Job drawing, mm, ordinate dimensions from the low corner. One solid piece. A direction names the side the tool comes from. Round coordinates to 2 decimals unless told otherwise and drop trailing zeros. Loops run counter-clockwise (first coordinate to the right, second up) from the corner with the lowest first, then second, coordinate; pieces in that order, holes last. Notation, with made-up numbers: M -37.75,-26 L -23.75,-26 A26 cw -23.75,13 Z; hole C 39,-40 d1. An arc over 180 degrees is marked long. One line per item, written item: value.
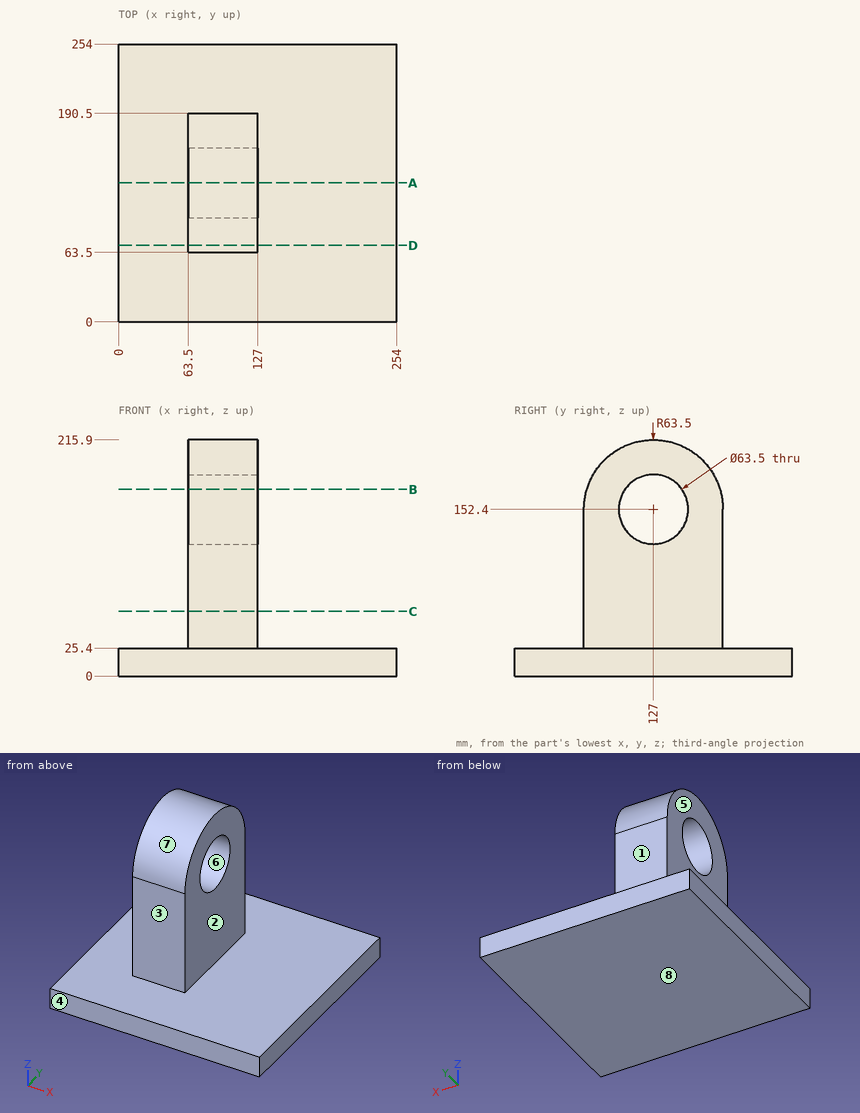
Item 1: Wall check: line 1 along Z through (x, y) = (89, 127); line 2 along Y through (x, z) = (83, 152); line 3 along X through (y, z) = (100.5, 58.5). Give the ranges that are in metal, low to high.
Check values:
line 1: z = 0 to 120.65, 184.15 to 215.9
line 2: y = 63.5 to 95.25, 158.75 to 190.5
line 3: x = 63.5 to 127
Item 2: Which spindle directions (+Z, -Z, +X, -X, +Y, -Y) get a long thin tool onto all of the face, cutting with end or side? Do the marked faces 1, 2, 3 and 4. Say none if no direction does.
Check values:
face 1: +Z, +X, -X, +Y
face 2: +Z, +X, +Y, -Y
face 3: +Z, +X, -X, -Y
face 4: +Z, -Z, +X, -X, -Y
Item 3: Slice it at A-A, the plane y = 127. Give the cut face in (x, z).
Check values:
outline: M 0,0 L 254,0 L 254,25.4 L 127,25.4 L 127,120.65 L 63.5,120.65 L 63.5,25.4 L 0,25.4 Z; M 63.5,184.15 L 127,184.15 L 127,215.9 L 63.5,215.9 Z
Item 4: Slice it at C-C, the plane z = 59. Give the cut face in (x, y), and give its area (3 significant figures).
Check values:
outline: M 63.5,63.5 L 127,63.5 L 127,190.5 L 63.5,190.5 Z
area: 8,060 mm2
Item 5: Drop flat-ended pins along their axis: P1, Ø2, axis at y = 171.5, z = 77.5, coming from the -X side; P2, Ø4, axis at y = 164.5, z = 161.5, coming from the +X side; P3, Ø6, axis at x = 42.5, y = 141, coming from the +Z side. Give the stop position or say it passes through.
Check values:
P1: stops at x = 63.5
P2: stops at x = 127
P3: stops at z = 25.4
Item 6: Slice it at B-B, the plane z = 170.5. Give the cut face in (x, y), and give its area (3 significant figures).
Check values:
outline: M 63.5,66.13 L 127,66.13 L 127,100.91 L 63.5,100.91 Z; M 63.5,153.09 L 127,153.09 L 127,187.87 L 63.5,187.87 Z
area: 4,420 mm2
Item 7: Pull direction Z, two halves, no side cores. Call the marked faces 5, 6, 7 and 8: pulls with the +Z half, pulls with the -Z half, needs draft (parallel to the pull), parting line crosses it, or undercut.
Check values:
face 5: needs draft
face 6: undercut
face 7: pulls with the +Z half
face 8: pulls with the -Z half
Item 8: Slice it at D-D, the plane y = 70. Give the cut face in (x, z).
Check values:
outline: M 0,0 L 254,0 L 254,25.4 L 127,25.4 L 127,180.39 L 63.5,180.39 L 63.5,25.4 L 0,25.4 Z
